```python
from build123d import *

# Parameters (mm, degrees)
F1_DEPTH = 3.175
F3_D     = 1.27


# Not quite as in the source:
# - a feature names something its author has since deleted; it is built from what else it names


with BuildPart() as f1:
    # F0 (on Front) → F1 (new body, symmetric)
    with BuildSketch(Plane.XZ):
        with BuildLine():
            Line((9.525, 59.69), (9.525, 63.5))
            Line((9.525, 63.5), (0, 63.5))
            Line((0, 63.5), (-9.525, 63.5))
            Line((-9.525, 63.5), (-9.525, 0))
            Line((-9.525, 0), (-0.635, 0))
            ThreePointArc((-0.635, 0), (0, 0.635), (0.635, 0))
            Line((0.635, 0), (9.525, 0))
            Line((9.525, 0), (9.525, 57.15))
            Line((9.525, 57.15), (7.9769473523, 57.15))
            Line((7.9769473523, 57.15), (7.9769473523, 59.69))
            Line((7.9769473523, 59.69), (9.525, 59.69))
        make_face()
        with BuildLine():
            ThreePointArc((0.635, 50.8), (-0.4490128061, 50.3509871939), (0, 51.435))
            ThreePointArc((0, 51.435), (0.4490128061, 51.2490128061), (0.635, 50.8))
        make_face(mode=Mode.SUBTRACT)
        with BuildLine():
            ThreePointArc((3.450873254, -8.8778994579), (7.861144724, -5.3784782818), (9.525, 0))
            Line((9.525, 0), (0.635, 0))
            ThreePointArc((0.635, 0), (0.5001354304, -0.3912665987), (0.1528281851, -0.6163347677))
            Line((0.1528281851, -0.6163347677), (1.3754536657, -5.5470129091))
            Line((1.3754536657, -5.5470129091), (3.450873254, -8.8778994579))
        make_face()
        with BuildLine():
            Line((-0.635, 0), (-9.525, 0))
            ThreePointArc((-9.525, 0), (-6.7351920908, -6.7351920908), (0, -9.525))
            Line((0, -9.525), (1.3754536657, -5.5470129091))
            Line((1.3754536657, -5.5470129091), (0.1528281851, -0.6163347677))
            ThreePointArc((0.1528281851, -0.6163347677), (-0.3912665987, -0.5001354304), (-0.635, 0))
        make_face()
    extrude(amount=F1_DEPTH, both=True)

    # F3 (through all)
    with Locations(Plane.YZ.offset(9.525)):
        with Locations((0, 58.42)):
            Hole(F3_D / 2)


solid = f1.part
```
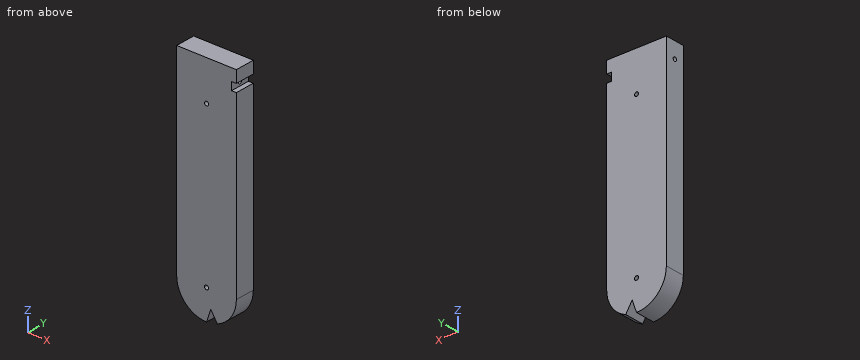
Work out the finished part from the listing and answer in its coordinate system (mm). Give positions to 0.01 mm unless a question says otherwise; leave off trailing zeros. Order: outer loops, then holes, each group sorted by start corner. A loop starts at its lowest first (then second) coordinate and runs counter-clockwise, first axis right, second up. Notation, with made-up numbers: M 38.5,-13.5 L 91.5,-13.5 A24 cw 91.5,-1.5 Z; hole C 59.5,-33 d10. An arc over 180 degrees is marked long. Return JSON: item names as keys, results as strings.
1) Section A-A, the plane z = 58.42 is taken. Write down the section's boundary in (x, y) (3 decimals), plus the area to 3 significant figures.
Resolved:
{"outline": "M -9.525,-3.175 L 7.977,-3.175 L 7.977,-0.635 L -9.525,-0.635 Z; M -9.525,0.635 L 7.977,0.635 L 7.977,3.175 L -9.525,3.175 Z", "area": "88.9 mm^2"}
2) Straight lines are drawn through the part: line 1 along X through (y, z) = (1.65, 50.8) (3 decimals); line 2 along Y through (x, z) = (-1.75, 58.42) (3 decimals); line 3 along Z through (x, y) = (2.75, 0) (3 decimals). For each, find the intervals that lie inside material, in ascending order. Write a range as [from, to].
Resolved:
{"line 1": "[-9.525, -0.635], [0.635, 9.525]", "line 2": "[-3.175, -0.635], [0.635, 3.175]", "line 3": "[-7.753, 57.785], [59.055, 63.5]"}
3) Each of these flat-tipped pins is pushed along its axis until it touches: pin 1 (3 mm diameter, centred on x = -5.5, y = 0, fed in from -Z); pin 2 (0.8 mm diameter, centred on x = 8.5, y = -1.5, fed in from -Z); pin 3 (1 mm diameter, centred on y = 0, z = 58.42, fed in from +X). Where does it stop, or does it pass through?
Resolved:
{"pin 1": "z = -8.64", "pin 2": "z = -5.01", "pin 3": "through"}
4) Section D-D, the plane z = -4 is taken. Write down the section's boundary in (x, y) (3 decimals).
Resolved:
{"outline": "M -8.644,-3.175 L 8.644,-3.175 L 8.644,3.175 L -8.644,3.175 Z"}
5) Section C-C, the plane x = 7 is taken. Write down the section's boundary in (y, z) (3 decimals).
Resolved:
{"outline": "M -3.175,-6.46 L 3.175,-6.46 L 3.175,63.5 L -3.175,63.5 Z; hole C 0,58.42 d1.27"}
6) Section B-B, the plane y = 1.25 is taken. Write down the section's boundary in (x, z) (3 decimals), plus the area to 3 significant figures.
Resolved:
{"outline": "M -9.525,0 A9.525 ccw 0,-9.525 L 1.375,-5.547 L 3.451,-8.878 A9.525 ccw 9.525,0 L 9.525,57.15 L 7.977,57.15 L 7.977,59.69 L 9.525,59.69 L 9.525,63.5 L -9.525,63.5 Z; hole C 0,0 d1.27; hole C 0,50.8 d1.27", "area": "1,340 mm^2"}
